Could you check a few things on this model? Use its own coordinates, in mm. Coordinates: 2 decimals unless noted, no trailing zeros. Loops run counter-clockwise (first coordinate to the right, second up) from the corner with the lowest first, then second, coordinate; pieces in that order, holes last. Notation, with made-up numbers: (15, 85) -> (22, 85) arc R11 cw to (22, 101) -> close; hole circle Ø6 at (-36, 3.5). An arc over 180 degrees is marked (long way). One line per question, with ' | ' between items.
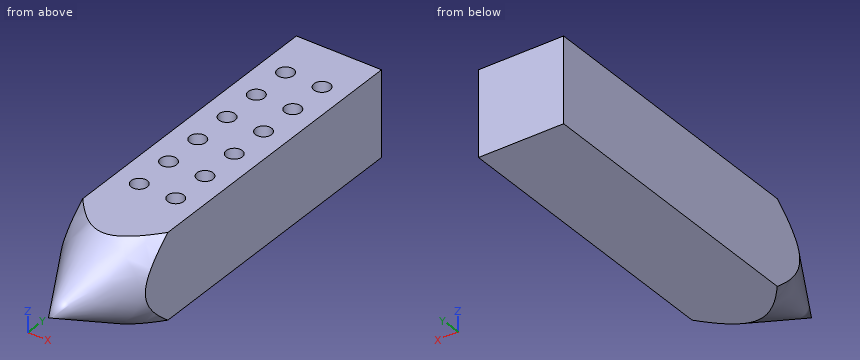
```python
from build123d import *

# Parameters (mm, degrees)
F0_W      = 42
F0_H      = 42
F1_DEPTH  = 146
F2_R      = 29.6984848098
F4_R      = 21
F5_DEPTH  = 25
F6_R      = 21
F9_DEPTH  = 25
F7_R      = 21
F10_DEPTH = 25
F8_R      = 21
F11_DEPTH = 25
F12_R     = 4
F13_DEPTH = 20


# Not quite as in the source:
# - an extrude whose draft closes it to a point is written as a loft to that point


with BuildPart() as f1:
    # F0 (on Front) → F1 (new body)
    with BuildSketch(Plane.XZ):
        Rectangle(F0_W, F0_H)
    extrude(amount=F1_DEPTH)

    # F2 (on face) → F3 section 0
    with BuildSketch(Plane.XZ.offset(146), mode=Mode.PRIVATE) as f3_s0:
        Circle(F2_R)
    loft([f3_s0.sketch, Vertex(0, -198.4999999927, 0)], ruled=True)

    # F4 (on face) → F5 (cut)
    with BuildSketch(Plane(origin=(-21, 0, 0), x_dir=(0, -1, 0), z_dir=(-1, 0, 0))):
        with Locations((146, 0)):
            Circle(F4_R)
    extrude(amount=F5_DEPTH, mode=Mode.SUBTRACT)

    # F6 (on face) → F9 (cut)
    with BuildSketch(Plane.XY.offset(21)):
        with Locations((0, -146)):
            Circle(F6_R)
    extrude(amount=F9_DEPTH, mode=Mode.SUBTRACT)

    # F7 (on face) → F10 (cut)
    with BuildSketch(Plane.YZ.offset(21)):
        with Locations((-146, 0)):
            Circle(F7_R)
    extrude(amount=F10_DEPTH, mode=Mode.SUBTRACT)

    # F8 (on face) → F11 (cut)
    with BuildSketch(Plane(origin=(0, 0, -21), x_dir=(1, 0, 0), z_dir=(0, 0, -1))):
        with Locations((0, 146)):
            Circle(F8_R)
    extrude(amount=F11_DEPTH, mode=Mode.SUBTRACT)

    # F12 (on face) → F13 (cut)
    with BuildSketch(Plane.XY.offset(21)):
        with Locations((-9, -24)):
            Circle(F12_R)
        with Locations((-9, -44)):
            Circle(F12_R)
        with Locations((-9, -64)):
            Circle(F12_R)
        with Locations((-9, -84)):
            Circle(F12_R)
        with Locations((-9, -104)):
            Circle(F12_R)
        with Locations((-9, -124)):
            Circle(F12_R)
        with Locations((9, -24)):
            Circle(F12_R)
        with Locations((9, -44)):
            Circle(F12_R)
        with Locations((9, -64)):
            Circle(F12_R)
        with Locations((9, -84)):
            Circle(F12_R)
        with Locations((9, -104)):
            Circle(F12_R)
        with Locations((9, -124)):
            Circle(F12_R)
    extrude(amount=-F13_DEPTH, mode=Mode.SUBTRACT)


solid = f1.part
```
Q1. Imagine slicing it at C-C on y = -179.5. Write out the boundary of the cut face in (x, z).
Values follow:
outline: circle Ø21.5 at (0, 0)
Q2. For pin 1 (4 mm diameter, centred on y = -176.5, z = -3, fed in from +X); pin 2 (6.5 mm diameter, centred on x = 8.5, y = -24, fed in from +Z), each with a flat end and sliding along its axis, tell me the tip position at first contact or that it passes through.
Values follow:
pin 1: stops at x = 13.31 | pin 2: stops at z = 1
Q3. Imagine slicing it at B-B on z = 14.5. Give the number of separate pieces and of enclosed holes in the cut face, plus the area to 3 significant figures.
Values follow:
separate pieces: 1 | enclosed holes: 12 | area: 6,350 mm2
Q4. Imagine slicing it at A-A on y = -84. Write out the boundary of the cut face in (x, z).
Values follow:
outline: (-21, -21) -> (21, -21) -> (21, 21) -> (13, 21) -> (13, 1) -> (5, 1) -> (5, 21) -> (-5, 21) -> (-5, 1) -> (-13, 1) -> (-13, 21) -> (-21, 21) -> close
